from build123d import *

# Parameters (mm, degrees)
SKETCH1_W           = 200.66
SKETCH1_H           = 99.06
BOSS_EXTRUDE1_DEPTH = 50.292
SKETCH2_W           = 12.7
SKETCH2_H           = 19.05
CUT_EXTRUDE1_DEPTH  = 213.713285349
SKETCH3_W           = 5.08
SKETCH3_H           = 12.7
CUT_EXTRUDE2_DEPTH  = 213.713285349
CUT_EXTRUDE3_DEPTH  = 213.713285349
BOSS_EXTRUDE2_DEPTH = 200.66
SKETCH6_W           = 12.7
SKETCH6_H           = 6.35
CUT_EXTRUDE4_DEPTH  = 213.713285349
CUT_EXTRUDE5_DEPTH  = 213.713285349
CUT_EXTRUDE6_DEPTH  = 5.08
BOSS_EXTRUDE3_DEPTH = 5.08
SKETCH13_W          = 152.4
SKETCH13_H          = 12.7
CUT_EXTRUDE7_DEPTH  = 2.54
FILLET1_R           = 6.35


with BuildPart() as part:
    # Sketch1 → Boss-Extrude1 (new body)
    with BuildSketch(Plane(origin=(0, 0, 0), x_dir=(1, 0, 0), z_dir=(0, 1, 0))):
        Rectangle(SKETCH1_W, SKETCH1_H)
    extrude(amount=-BOSS_EXTRUDE1_DEPTH)

    # Sketch2 → Cut-Extrude1 (cut, through all)
    with BuildSketch(Plane.ZY.offset(100.33)):
        with Locations((-30.48, -9.525)):
            Rectangle(SKETCH2_W, SKETCH2_H)
    cut_extrude1 = extrude(amount=-CUT_EXTRUDE1_DEPTH, mode=Mode.SUBTRACT)

    # Sketch3 → Cut-Extrude2 (cut, through all)
    with BuildSketch(Plane.ZY.offset(100.33)):
        with Locations((-26.67, -25.4)):
            Rectangle(SKETCH3_W, SKETCH3_H)
    cut_extrude2 = extrude(amount=-CUT_EXTRUDE2_DEPTH, mode=Mode.SUBTRACT)

    # Sketch4 → Cut-Extrude3 (cut, through all)
    with BuildSketch(Plane.ZY.offset(100.33)):
        Polygon((-24.13, -19.05), (-8.145152026, 0), (-24.13, 0), align=None)
    cut_extrude3 = extrude(amount=-CUT_EXTRUDE3_DEPTH, mode=Mode.SUBTRACT)

    # Mirror1: Cut-Extrude1, Cut-Extrude2, Cut-Extrude3 across plane
    add(cut_extrude1.mirror(Plane.XY), mode=Mode.SUBTRACT)
    add(cut_extrude2.mirror(Plane.XY), mode=Mode.SUBTRACT)
    add(cut_extrude3.mirror(Plane.XY), mode=Mode.SUBTRACT)

    # Sketch5 → Boss-Extrude2 (add)
    with BuildSketch(Plane(origin=(100.33, 0, 0), x_dir=(0, 0, -1), z_dir=(1, 0, 0))):
        Polygon((-24.13, -19.05), (-8.145152026, 0), (-24.13, 0), align=None)
    extrude(amount=-BOSS_EXTRUDE2_DEPTH)

    # Sketch6 → Cut-Extrude4 (cut, through all)
    with BuildSketch(Plane(origin=(100.33, 0, 0), x_dir=(0, 0, -1), z_dir=(1, 0, 0))):
        with Locations((0, -47.117)):
            Rectangle(SKETCH6_W, SKETCH6_H)
    extrude(amount=-CUT_EXTRUDE4_DEPTH, mode=Mode.SUBTRACT)

    # Sketch7 → Cut-Extrude5 (cut, through all)
    with BuildSketch(Plane.ZY.offset(100.33)):
        Polygon((24.13, -50.292), (24.13, -43.942), (36.83, -43.942), (47.828522628, -50.292), align=None)
    extrude(amount=-CUT_EXTRUDE5_DEPTH, mode=Mode.SUBTRACT)

    # Sketch8 → Cut-Extrude6 (cut)
    with BuildSketch(Plane.XY.offset(49.53)):
        with BuildLine():
            Line((-100.33, -18.542), (-100.33, -31.242))
            ThreePointArc((-100.33, -31.242), (0, -18.662836295), (100.33, -31.242))
            Line((100.33, -31.242), (100.33, -18.542))
            ThreePointArc((100.33, -18.542), (0, -5.962836295), (-100.33, -18.542))
        make_face()
    cut_extrude6 = extrude(amount=-CUT_EXTRUDE6_DEPTH, mode=Mode.SUBTRACT)

    # Mirror2: Cut-Extrude6 across plane
    add(cut_extrude6.mirror(Plane.XY), mode=Mode.SUBTRACT)

    # Sketch9 → Boss-Extrude3 (add)
    with BuildSketch(Plane(origin=(0, 0, -49.53), x_dir=(-1, 0, 0), z_dir=(0, 0, -1))):
        with BuildLine():
            Line((100.33, -18.542), (100.33, -31.242))
            ThreePointArc((100.33, -31.242), (50.5577498, -21.819889754), (0, -18.662836295))
            ThreePointArc((0, -18.662836295), (6.35, -12.312836295), (0, -5.962836295))
            ThreePointArc((0, -5.962836295), (50.5577498, -9.119889754), (100.33, -18.542))
        make_face()
    extrude(amount=-BOSS_EXTRUDE3_DEPTH)

    # Sketch13 → Cut-Extrude7 (cut)
    with BuildSketch(Plane(origin=(0, 0, 0), x_dir=(1, 0, 0), z_dir=(0, 1, 0))):
        with Locations((-100.33, -7.992423987)):
            Rectangle(SKETCH13_W, SKETCH13_H)
    extrude(amount=-CUT_EXTRUDE7_DEPTH, mode=Mode.SUBTRACT)

    # Fillet1
    fillet1_edges = [part.edges().sort_by_distance(p)[0] for p in [
        (-24.13, -1.27, 14.342423987),
        (-24.13, -1.27, 1.642423987),
    ]]
    fillet(fillet1_edges, radius=FILLET1_R - 0.0001)  # a hair under: the kernel refuses the full size


solid = part.part
Verification items for the finished model (mm, model axes). A direction names the side the tool comes from. Round coordinates to 2 decimals unless told otherwise and drop trailing zeros. Loops run counter-clockwise (first coordinate to the right, second up) from the corner with the lowest first, then second, coordinate; pieces in that order, holes last. Notation, with made-up numbers: (77, 46.25) - (131, 46.25) arc R13 cw to (131, 68.25) - close; hole circle Ø10 at (77.25, -14.75). An arc over 180 degrees is marked (long way). Answer in a Markdown table with one row per item. Add a question column.
Q1. Section check B-B on z = -2.5. Enter the section's corners in (x, y), plus the area to 3 significant figures.
Q2. Gauge pin test, flat ends, axial feed: pin 1 (5.5 mm diameter, centred on x = -41.5, y = -13.5, fed in from +Z); pin 2 (2.5 mm diameter, centred on x = 41.5, z = -35, fed in from +Y); pin 3 (4 mm diameter, centred on x = 8.5, z = -26.5, fed in from +Y). Record the tip position at first contact, or that the pin passes through.
Q3. Tool access check on faces 1 (the face through (51.26, -9.21, -47.03)), 2 (the face through (1, -43.942, 0)), 3 (the face through (-26.04, -1.29, 12.53)), 4 (the face through (-1, -10, -36.83)). Record the directions out of +Z, -Z, +X, -X, +Y, -Y that give a thin tool (end or side, any length) a straight path to the whole face; none if there is none.
Q4. Release check for a two-part mould opening along X. For faces 5 (the face through (1.419, -5.965, 47.026)), 6 (the face through (-1, -25, 29.21)), 7 (the face through (-100.33, -25, -1)) record: pulls with the +X half, pulls with the -X half, needs draft (parallel to the pull), parting line crosses it, or undercut.
Q5. Material ranges on line 1 (Z direction, x = 8.5, y = -29.5); line 2 (Z direction, x = 74, y = -22); line 3 (Y direction, x = -50, z = -2.5), recorded low to high.
Found:
| question | item | result |
|---|---|---|
| 1 | outline | (-100.33, -43.94) - (100.33, -43.94) - (100.33, 0) - (-100.33, 0) - close |
| 1 | area | 8,820 mm² |
| 2 | pin 1 | stops at z = 44.45 |
| 2 | pin 2 | stops at y = -19.05 |
| 2 | pin 3 | stops at y = -31.75 |
| 3 | face 1 | -Z |
| 3 | face 2 | +X, -X, -Y |
| 3 | face 3 | -X, +Y |
| 3 | face 4 | +X, -X, +Y |
| 4 | face 5 | undercut |
| 4 | face 6 | needs draft |
| 4 | face 7 | pulls with the -X half |
| 5 | line 1 | z = -49.53 to -29.21, -24.13 to 24.13, 29.21 to 49.53 |
| 5 | line 2 | z = -44.45 to -29.21, -24.13 to 24.13, 29.21 to 44.45 |
| 5 | line 3 | y = -43.94 to 0 |
